Verification items for this drawing (mm, ordinates from the low corner). Round coordinates to 2 decimals unless told otherwise and drop trailing zeros. Loops run counter-clockwise (first coordinate to the right, second up) from the corner with the lowest first, then second, coordinate; pieces in that order, holes last. Notation, with made-up numbers: (22.25, 15.25) - (67.25, 15.25) arc R25 ccw to (67.25, 48.25) - close; hole circle Ø9 at (48.25, 39). An arc over 180 degrees is marked (long way). Put each result on its own line as item: value.
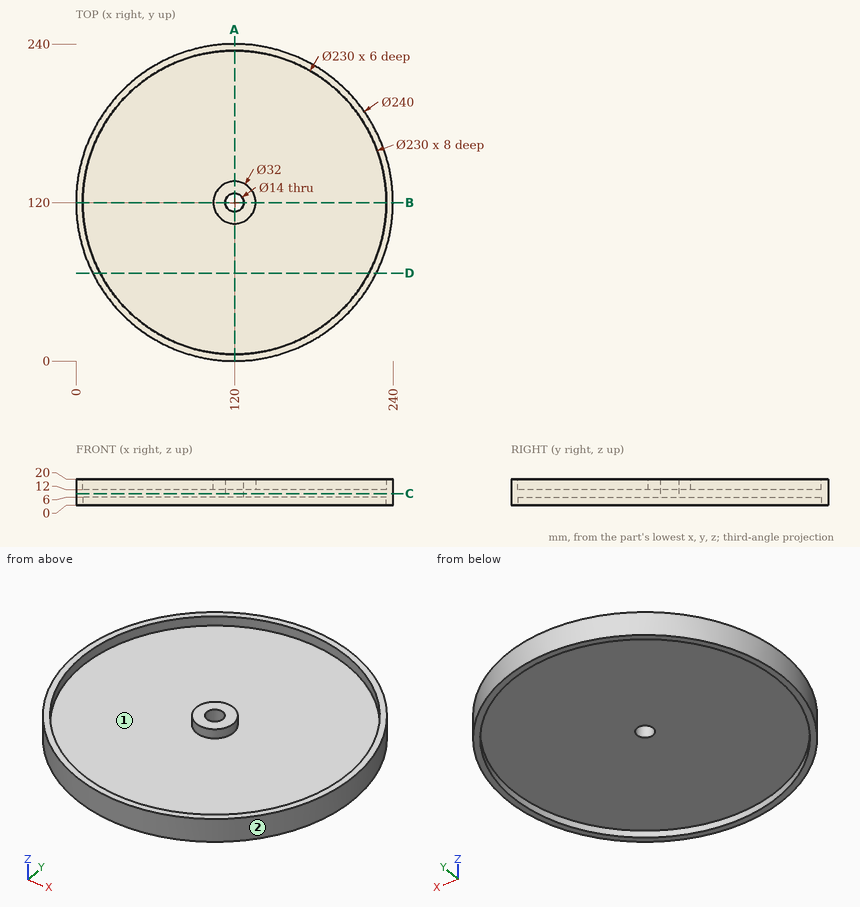
Item 1: Section check A-A on x = 120. Enter the section's corners in (y, z), then the cut area to 3 significant figures.
Filled sheet:
outline: (0, 0) - (5, 0) - (5, 6) - (113, 6) - (113, 20) - (104, 20) - (104, 12) - (5, 12) - (5, 20) - (0, 20) - close; (127, 6) - (235, 6) - (235, 0) - (240, 0) - (240, 20) - (235, 20) - (235, 12) - (136, 12) - (136, 20) - (127, 20) - close
area: 1,640 mm²
Item 2: Thickness scan on line 1 (Y direction, x = 120, z = 13.5); line 2 (Y direction, x = 120, z = 1.45); line 3 (Y direction, x = 120, z = 10.75). Record the ranges inside material, lowest first. Write a range as from..to.
Filled sheet:
line 1: 0..5, 104..113, 127..136, 235..240
line 2: 0..5, 235..240
line 3: 0..113, 127..240
Item 3: Section check D-D on y = 66.5. Enter the section's corners in (x, z), then the cut area to 3 significant figures.
Filled sheet:
outline: (12.59, 0) - (18.2, 0) - (18.2, 6) - (221.8, 6) - (221.8, 0) - (227.41, 0) - (227.41, 20) - (221.8, 20) - (221.8, 12) - (18.2, 12) - (18.2, 20) - (12.59, 20) - close
area: 1,450 mm²
Item 4: Release check for a two-part mould opening along X. For the marked faces 1 and 2 record: +X half, -X half, draft (parallel to the pull), parting line (faces both ways), or undercut.
Filled sheet:
face 1: undercut
face 2: parting line
Item 5: Go/stop test with flat-tipped pins: pin 1 (5 mm diameter, centred on x = 26, z = 4, fed in from +Y); pin 2 (6 mm diameter, centred on x = 206, y = 77.5, fed in from -Z); pin 3 (4 mm diameter, centred on y = 138.5, z = 17, fed in from +X). Record where each tip stops, or that it passes through.
Filled sheet:
pin 1: y = 197.64
pin 2: z = 6
pin 3: x = 238.86
Item 6: Section check C-C on z = 9. Enter the section's corners in (x, y).
Filled sheet:
outline: circle Ø240 at (120, 120); hole circle Ø14 at (120, 120)
